For this review, take the finished solid that the model builds, in its own axes (mm). A direction names the side the tool comes from. Round coordinates to 2 decimals unless told otherwise and drop trailing zeros. Order: outer loops, then holes, each group sorted by start corner. A loop starts at its lowest first (then second) coordinate and runs counter-clockwise, first axis right, second up. Notation, with made-up numbers: (44.5, 14.5) -> (93.5, 14.5) arc R4 cw to (93.5, 18.5) -> close; hole circle Ø5 at (-6.75, 86). An arc over 180 degrees is marked (long way). Answer in a Markdown table with one row per item.
Autodesk Inventor part; units mm, degrees
ref_plane "YZ Plane" through (0, 0, 0) normal (1, 0, 0) x (0, 1, 0)
ref_plane "XZ Plane" through (0, 0, 0) normal (0, 1, 0) x (-1, 0, 0)
ref_plane "XY Plane" through (0, 0, 0) normal (0, 0, 1) x (1, 0, 0)
sketch "Sketch1" plane through (0, 0, 0) normal (0, 1, 0) x (-1, 0, 0)
  line L0 (0, 0) -> (58, 0)
  line L1 (58, 0) -> (58, -50)
  line L2 (58, -50) -> (0, -50)
  line L3 (0, -50) -> (0, 0)
  line L4 (0, -50) -> (50, -50)
  line L5 (50, -50) -> (50, -23)
  line L6 (35, -8) -> (0, -8)
  line L7 (0, -8) -> (0, -50)
  arc A0 (50, -23) -> (35, -8) centre (35, -23) ccw
  line L8 (54, -53.5159) -> (54, 28.6039) construction
  line L9 (-7.6056, -4) -> (76.8297, -4) construction
  point P0 (50, -8)
  point P1 (6, -4)
  point P2 (18, -4)
  point P3 (54, -32)
  point P4 (54, -44)
  point P5 (50, -8)
  dimension "d0" = 58
  dimension "d1" = 50
  dimension "d2" = 50
  dimension "d3" = 42
  dimension "d4" = 15
  dimension "d5" = 6
  dimension "d6" = 18
  dimension "d7" = 18
  dimension "d8" = 6
extrude "Extrusion1" add sketch "Sketch1" against normal blind 5 contours L0 L1 L2 L5 A0 L6 L3
hole "Hole1" at (-6, 0, -4) at (-18, 0, -4) at (-54, 0, -32) at (-54, 0, -44) at (-50, 0, -8) direction (0, -1, 0) diameter 3.8 end through all
properties part number "Step-back spacer -electronics enc"
Q1. To check wall thickness, follow probe 1 along Z at (x, y) = (-54, -1.3); probe 2 along X at (y, z) = (-2.9, -44); probe 3 along X at (y, z) = (-1.2, -24). State the ranges of each line that lie inside material, in increasing order.
Answer key:
| item | result |
|---|---|
| probe 1 | z = -50 to -45.9, -42.1 to -33.9, -30.1 to 0 |
| probe 2 | x = -58 to -55.9, -52.1 to -50 |
| probe 3 | x = -58 to -50 |
Q2. Take a section at B-B, the plane x = -54. Write out the cut boundary in (y, z), then the cut area to 3 significant figures.
Answer key:
| item | result |
|---|---|
| outline | (-5, -50) -> (0, -50) -> (0, -45.9) -> (-5, -45.9) -> close; (-5, -42.1) -> (0, -42.1) -> (0, -33.9) -> (-5, -33.9) -> close; (-5, -30.1) -> (0, -30.1) -> (0, 0) -> (-5, 0) -> close |
| area | 212 mm^2 |
Q3. Tool access review of faces 1 (the face through (-19.884, -2.535, -4.247)), 2 (the face through (-50, -2, -37)): name each direction out of +Z, -Z, +X, -X, +Y, -Y from which nothing blocks a thin tool from reaching the whole face with its end or side.
Answer key:
| item | result |
|---|---|
| face 1 | +Y, -Y |
| face 2 | -Z, +X, +Y, -Y |
Q4. Clearance check with flat-ended pins moving along their axes: pin 1 Ø1 at (y, z) = (-3.5, -29.5) entering from +X; pin 2 Ø1 at (x, y) = (-29, -1.5) entering from -Z. State where each tip first meets the part, or that it passes through.
Answer key:
| item | result |
|---|---|
| pin 1 | stops at x = -50 |
| pin 2 | stops at z = -8 |
Q5. Take a section at D-D, the plane z = -32. Write out the cut boundary in (x, y), then the cut area to 3 significant figures.
Answer key:
| item | result |
|---|---|
| outline | (-58, -5) -> (-55.9, -5) -> (-55.9, 0) -> (-58, 0) -> close; (-52.1, -5) -> (-50, -5) -> (-50, 0) -> (-52.1, 0) -> close |
| area | 21.0 mm^2 |
Q6. Take a section at C-C, the plane y = -1.55. Write out the cut boundary in (x, z), then the cut area to 3 significant figures.
Answer key:
| item | result |
|---|---|
| outline | (-58, -50) -> (-50, -50) -> (-50, -23) arc R15 cw to (-35, -8) -> (0, -8) -> (0, 0) -> (-58, 0) -> close; hole circle Ø3.8 at (-54, -44); hole circle Ø3.8 at (-54, -32); hole circle Ø3.8 at (-50, -8); hole circle Ø3.8 at (-18, -4); hole circle Ø3.8 at (-6, -4) |
| area | 792 mm^2 |
Q7. Take a section at A-A, the plane z = -4. Write out the cut boundary in (x, y).
Answer key:
| item | result |
|---|---|
| outline | (-58, -5) -> (-19.9, -5) -> (-19.9, 0) -> (-58, 0) -> close; (-16.1, -5) -> (-7.9, -5) -> (-7.9, 0) -> (-16.1, 0) -> close; (-4.1, -5) -> (0, -5) -> (0, 0) -> (-4.1, 0) -> close |
Q8. The part is to be moulded in two halves that separate along Z. For faces 3 (the face through (-58, -2, -25)), 4 (the face through (-29, -2, 0)), 5 (the face through (-52.314, -2.535, -43.123)), say which applies: +Z half, -Z half, draft (parallel to the pull), parting line (faces both ways), or undercut.
Answer key:
| item | result |
|---|---|
| face 3 | draft |
| face 4 | +Z half |
| face 5 | undercut |
